Here's the drawing with two shaded views (mm, measured from the low corner). I have some questions. Round coordinates to 2 decimals unless told otherwise and drop trailing zeros. Loops run counter-clockwise (first coordinate to the right, second up) from the corner with the lowest first, then second, coordinate; pieces in that order, holes last. Notation, with made-up numbers: (-16.75, -31) -> (-10.75, -31) arc R22 ccw to (-10.75, 7) -> close; hole circle Ø11 at (82, 80.25). An arc over 180 degrees is marked (long way). Use a Markdown table: item, result.
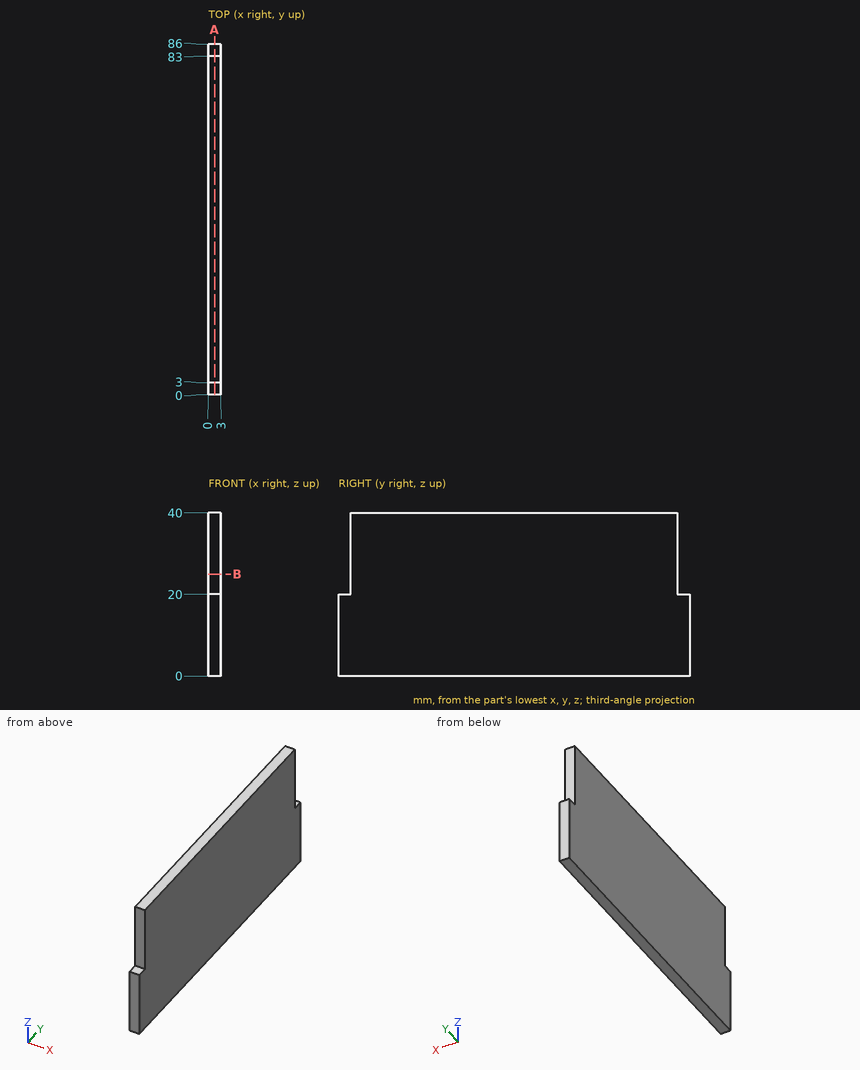
1. Will these pins go through, and if not, where does the flat tip stop? pin 1 Ø1.5 at (x, y) = (1, 84) entering from +Z; pin 2 Ø0.9 at (x, z) = (1, 33) entering from +Y; pin 3 Ø1.5 at (x, z) = (0.5, 26) entering from -Y.
Answer sheet:
| item | result |
|---|---|
| pin 1 | stops at z = 20 |
| pin 2 | stops at y = 83 |
| pin 3 | stops at y = 3 |
2. I need wall thicknesses on line 1 (Y direction, x = 1.2, z = 27). Which ranges of the line are inside material? Lowest first, please.
Answer sheet:
| item | result |
|---|---|
| line 1 | y = 3 to 83 |
3. I want a section at A-A (x = 1.5). Please give me the cut outline in (y, z), plus the area to 3 significant figures.
Answer sheet:
| item | result |
|---|---|
| outline | (0, 0) -> (86, 0) -> (86, 20) -> (83, 20) -> (83, 40) -> (3, 40) -> (3, 20) -> (0, 20) -> close |
| area | 3,320 mm² |
4. I want a section at B-B (z = 25). Please give me the cut outline in (x, y).
Answer sheet:
| item | result |
|---|---|
| outline | (0, 3) -> (3, 3) -> (3, 83) -> (0, 83) -> close |
